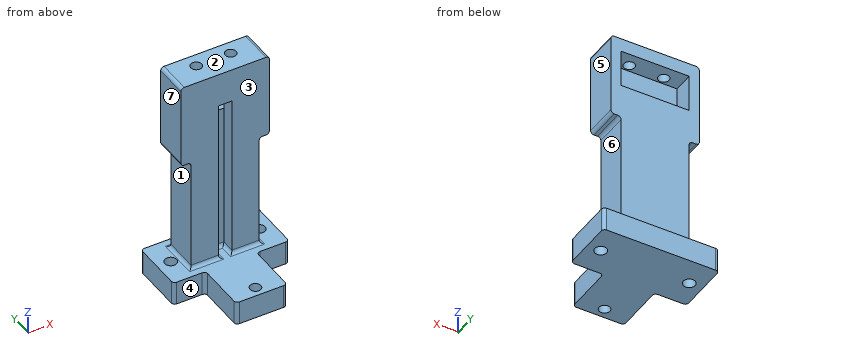
```python
from build123d import *

# Parameters (mm, degrees)
SKETCH_W           = 20
SKETCH_H           = 10
PAD_DEPTH          = 60
SKETCH001_W        = 50
SKETCH001_H        = 10
PAD001_DEPTH       = 10
PAD001_FACE6_W     = 10
PAD001_FACE6_H     = 15
PAD002_DEPTH       = 5
PAD002_FACE5_W     = 10
PAD002_FACE5_H     = 15
PAD003_DEPTH       = 5
SKETCH002_W        = 20
SKETCH002_H        = 11
POCKET_DEPTH       = 6
PAD004_DEPTH       = 10
PAD005_DEPTH       = 10
PAD005_FACE15_W    = 10
PAD005_FACE15_H    = 25
POCKET001_DEPTH    = 12
POCKET001_FACE3_W  = 10
POCKET001_FACE3_H  = 25
POCKET002_DEPTH    = 12
SKETCH003_W        = 4
SKETCH003_H        = 56
POCKET003_DEPTH    = 4
SKETCH004_R        = 1.6
POCKET004_DEPTH    = 30
SKETCH005_W        = 30
SKETCH005_H        = 12
PAD006_DEPTH       = 7
SKETCH006_R        = 1.75
POCKET005_DEPTH    = 9
POCKET005_FACE23_W = 12
POCKET005_FACE23_H = 7
PAD007_DEPTH       = 2
PAD007_FACE1_W     = 12
PAD007_FACE1_H     = 7
PAD008_DEPTH       = 2
FILLET_R           = 1
FILLET_FACE10_W    = 34
FILLET_FACE10_H    = 7
PAD009_DEPTH       = 2
PAD009_FACE3_W     = 34
PAD009_FACE3_H     = 7
PAD010_DEPTH       = 2
FILLET001_R        = 1
FILLET002_R        = 1
FILLET003_R        = 1
SKETCH007_W        = 15
SKETCH007_H        = 7
PAD011_DEPTH       = 15
FILLET004_R        = 1
SKETCH008_R        = 1.6
POCKET006_DEPTH    = 10


with BuildPart() as part:
    # Sketch → Pad (new body)
    with BuildSketch(Plane.XY):
        Rectangle(SKETCH_W, SKETCH_H)
    extrude(amount=PAD_DEPTH)

    # Sketch001 (on Face2 of Pad) → Pad001 (join)
    with BuildSketch(Plane.XZ.offset(5)):
        with Locations((0, 61)):
            Rectangle(SKETCH001_W, SKETCH001_H)
    extrude(amount=-PAD001_DEPTH)

    # Pad001 Face6 → Pad002 (add)
    with BuildSketch(Plane(origin=(17.5, 0, 56), x_dir=(0, -1, 0), z_dir=(0, 0, -1))):
        Rectangle(PAD001_FACE6_W, PAD001_FACE6_H)
    extrude(amount=PAD002_DEPTH)

    # Pad002 Face5 → Pad003 (add)
    with BuildSketch(Plane(origin=(-17.5, 0, 56), x_dir=(0, -1, 0), z_dir=(0, 0, -1))):
        Rectangle(PAD002_FACE5_W, PAD002_FACE5_H)
    extrude(amount=PAD003_DEPTH)

    # Sketch002 (on Face10 of Pad003) → Pocket (cut)
    with BuildSketch(Plane(origin=(0, 5, 0), x_dir=(-1, 0, 0), z_dir=(0, 1, 0))):
        with Locations((0, 56.5)):
            Rectangle(SKETCH002_W, SKETCH002_H)
    extrude(amount=-POCKET_DEPTH, mode=Mode.SUBTRACT)

    # Pocket Face6 → Pad004 (add)
    with BuildSketch(Plane(origin=(-17.5, 0, 51), x_dir=(0, -1, 0), z_dir=(0, 0, -1))):
        Polygon((5, -7.5), (5, 7.5), (-5, 7.5), (-5, -7.5), (1, -7.5), align=None)
    extrude(amount=PAD004_DEPTH)

    # Pad004 Face5 → Pad005 (add)
    with BuildSketch(Plane(origin=(17.5, 0, 51), x_dir=(0, -1, 0), z_dir=(0, 0, -1))):
        Polygon((5, -7.5), (5, 7.5), (1, 7.5), (-5, 7.5), (-5, -7.5), align=None)
    extrude(amount=PAD005_DEPTH)

    # Pad005 Face15 → Pocket001 (cut)
    with BuildSketch(Plane(origin=(25, 0, 53.5), x_dir=(0, -1, 0), z_dir=(1, 0, 0))):
        Rectangle(PAD005_FACE15_W, PAD005_FACE15_H)
    extrude(amount=-POCKET001_DEPTH, mode=Mode.SUBTRACT)

    # Pocket001 Face3 → Pocket002 (cut)
    with BuildSketch(Plane(origin=(-25, 0, 53.5), x_dir=(0, 1, 0), z_dir=(-1, 0, 0))):
        Rectangle(POCKET001_FACE3_W, POCKET001_FACE3_H)
    extrude(amount=-POCKET002_DEPTH, mode=Mode.SUBTRACT)

    # Sketch003 (on Face2 of Pocket002) → Pocket003 (cut)
    with BuildSketch(Plane.XZ.offset(5)):
        with Locations((0, 28)):
            Rectangle(SKETCH003_W, SKETCH003_H)
    extrude(amount=-POCKET003_DEPTH, mode=Mode.SUBTRACT)

    # Sketch004 (on Face1 of Pocket003) → Pocket004 (cut)
    with BuildSketch(Plane.XY.offset(66)):
        with Locations((-4.9, 1)):
            Circle(SKETCH004_R)
        with Locations((5.2, 1)):
            Circle(SKETCH004_R)
    extrude(amount=-POCKET004_DEPTH, mode=Mode.SUBTRACT)

    # Sketch005 (on Face12 of Pocket004) → Pad006 (join)
    with BuildSketch(Plane(origin=(0, 0, 0), x_dir=(1, 0, 0), z_dir=(0, 0, -1))):
        Rectangle(SKETCH005_W, SKETCH005_H)
    extrude(amount=-PAD006_DEPTH)

    # Sketch006 (on Face12 of Pad006) → Pocket005 (cut)
    with BuildSketch(Plane.XY.offset(7)):
        with Locations((13, 0)):
            Circle(SKETCH006_R)
        with Locations((-13, 0)):
            Circle(SKETCH006_R)
    extrude(amount=-POCKET005_DEPTH, mode=Mode.SUBTRACT)

    # Pocket005 Face23 → Pad007 (add)
    with BuildSketch(Plane(origin=(15, 0, 3.5), x_dir=(0, -1, 0), z_dir=(1, 0, 0))):
        Rectangle(POCKET005_FACE23_W, POCKET005_FACE23_H)
    extrude(amount=PAD007_DEPTH)

    # Pad007 Face1 → Pad008 (add)
    with BuildSketch(Plane(origin=(-15, 0, 3.5), x_dir=(0, 1, 0), z_dir=(-1, 0, 0))):
        Rectangle(PAD007_FACE1_W, PAD007_FACE1_H)
    extrude(amount=PAD008_DEPTH)

    # Fillet
    fillet_edges = [part.edges().sort_by_distance(p)[0] for p in [
        (0, -1, 7),
        (-2, -3, 7),
        (2, -3, 7),
    ]]
    fillet(fillet_edges, radius=FILLET_R)

    # Fillet Face10 → Pad009 (add)
    with BuildSketch(Plane(origin=(0, 6, 3.5), x_dir=(1, 0, 0), z_dir=(0, 1, 0))):
        Rectangle(FILLET_FACE10_W, FILLET_FACE10_H)
    extrude(amount=PAD009_DEPTH)

    # Pad009 Face3 → Pad010 (add)
    with BuildSketch(Plane(origin=(0, -6, 3.5), x_dir=(-1, 0, 0), z_dir=(0, -1, 0))):
        Rectangle(PAD009_FACE3_W, PAD009_FACE3_H)
    extrude(amount=PAD010_DEPTH)

    # Fillet001
    fillet001_edges = [part.edges().sort_by_distance(p)[0] for p in [
        (0, 5, 7),
        (-10, 0, 7),
        (10, 0, 7),
        (5.5, -5, 7),
        (-5.5, -5, 7),
    ]]
    fillet(fillet001_edges, radius=FILLET001_R)

    # Fillet002
    fillet002_edges = [part.edges().sort_by_distance(p)[0] for p in [
        (10, 0, 41),
        (13, 0, 41),
        (-10, 0, 41),
        (-13, 0, 41),
    ]]
    fillet(fillet002_edges, radius=FILLET002_R)

    # Fillet003
    fillet003_edges = [part.edges().sort_by_distance(p)[0] for p in [
        (-13, 0, 66),
        (13, 0, 66),
        (-17, 8, 3.5),
        (-17, -8, 3.5),
        (17, 8, 3.5),
        (17, -8, 3.5),
    ]]
    fillet(fillet003_edges, radius=FILLET003_R)

    # Sketch007 (on Face42 of Fillet003) → Pad011 (join)
    with BuildSketch(Plane.XZ.offset(8)):
        with Locations((0, 3.5)):
            Rectangle(SKETCH007_W, SKETCH007_H)
    extrude(amount=PAD011_DEPTH)

    # Fillet004
    fillet004_edges = [part.edges().sort_by_distance(p)[0] for p in [
        (-7.5, -23, 3.5),
        (7.5, -23, 3.5),
        (-7.5, -8, 3.5),
        (7.5, -8, 3.5),
    ]]
    fillet(fillet004_edges, radius=FILLET004_R)

    # Sketch008 (on Face5 of Fillet004) → Pocket006 (cut)
    with BuildSketch(Plane.XY.offset(7)):
        with Locations((0, -20)):
            Circle(SKETCH008_R)
    extrude(amount=-POCKET006_DEPTH, mode=Mode.SUBTRACT)


solid = part.part
```
Part model, mm, in its own coordinate system. Face numbers are marked on the shaded views. A direction names the side the tool comes from. Coordinates: 2 decimals unless noted, no trailing zeros. Order: outer loops, then holes, each group sorted by start corner. A loop starts at its lowest first (then second) coordinate and runs counter-clockwise, first axis right, second up. Notation, with made-up numbers: (1, 38) - (43, 38) arc R11 ccw to (43, 52) - close; hole circle Ø9 at (25, 39). An arc over 180 degrees is marked (long way). Return JSON: item names as keys, results as strings. Group by question number.
Item 1: Cut at C-C (x = -4.9). List the corners of the cut face in (y, z), plus the area to 3 significant figures.
Item 2: Drill centre lines: probe 1 along Y at (x, z) = (0, 3.5); probe 2 along Y at (x, z) = (-4.9, 45.75); probe 3 along Z at (x, y) = (3.5, -14). Where is each one in solid material? Low to high. Write a range as from..to.
Item 3: Pull direction Z, two halves, no side cores. Call the marked faces 1, 2 and 3: pulls with the +Z half, pulls with the -Z half, needs draft (parallel to the pull), parting line crosses it, or undercut.
Item 4: Cut at D-D (z = 15). List the corners of the cut face in (x, y).
Item 5: Which spindle directions (+Z, -Z, +X, -X, +Y, -Y) get a long thin tool onto all of the face, cutting with end or side? Do the marked faces 4, 5, 6 and 7. Say none if no direction does.
Item 6: Cut at B-B (y = -20). List the corners of the cut face in (x, z).
Item 7: Cut at A-A (x = 0). List the corners of the cut face in (y, z).
Item 8: Pin check, flat tips, straight feed: pin 1 (12 mm diameter, centred on x = -4, z = 57.5, fed in from +Y); pin 2 (7.5 mm diameter, centred on x = 12.5, z = 4, fed in from -Y); pin 3 (3.5 mm diameter, centred on y = -18.5, z = 4.5, fed in from -X). Stop position of each tip, or through.
Check values:
{
 "1": {"outline": "(-23, 0) - (8, 0) - (8, 7) - (6, 7) arc R1 cw to (5, 8) - (5, 51) - (2.6, 51) - (2.6, 36) - (-0.6, 36) - (-0.6, 51) - (-1, 51) - (-1, 62) - (-0.6, 62) - (-0.6, 66) - (-5, 66) - (-5, 8) arc R1 cw to (-6, 7) - (-23, 7) - close; (2.6, 62) - (5, 62) - (5, 66) - (2.6, 66) - close", "area": "681 mm2"},
 "2": {"probe 1": "y = -23..-21.6, -18.4..8", "probe 2": "y = -5..-0.6, 2.6..5", "probe 3": "z = 0..7"},
 "3": {"face 1": "undercut", "face 2": "pulls with the +Z half", "face 3": "needs draft"},
 "4": {"outline": "(-10, -5) - (-2, -5) - (-2, -1) - (2, -1) - (2, -5) - (10, -5) - (10, 5) - (-10, 5) - close"},
 "5": {"face 4": "+Z, -Z, -X, -Y", "face 5": "+Z, +X, +Y, -Y", "face 6": "+X, +Y, -Y", "face 7": "+Z, -X, +Y, -Y"},
 "6": {"outline": "(-7.5, 0) - (-1.6, 0) - (-1.6, 7) - (-7.5, 7) - close; (1.6, 0) - (7.5, 0) - (7.5, 7) - (1.6, 7) - close"},
 "7": {"outline": "(-23, 0) - (-21.6, 0) - (-21.6, 7) - (-23, 7) - close; (-18.4, 0) - (8, 0) - (8, 7) - (6, 7) arc R1 cw to (5, 8) - (5, 51) - (-1, 51) - (-1, 8) arc R1 cw to (-2, 7) - (-18.4, 7) - close; (-5, 56) - (-1, 56) - (-1, 62) - (5, 62) - (5, 66) - (-5, 66) - close"},
 "8": {"pin 1": "stops at y = 5", "pin 2": "stops at y = -8", "pin 3": "stops at x = -7.5"}
}
